from build123d import *

# Parameters (mm, degrees)
F0_W     = 47.625
F0_H     = 19.05
F1_DEPTH = 63.5
F0_W_2   = 25.4
F2_DEPTH = 25.4
F3_DEPTH = 7.9375


# Not quite as in the source:
# - a feature of the source that left no trace in its solid (it failed there, or was rolled back) is left out


with BuildPart() as f1:
    # F0 (on Front) → F1 (new body, symmetric)
    with BuildSketch(Plane.XZ):
        with Locations((-23.8125, 0)):
            Rectangle(F0_W, F0_H)
        Polygon((28.575, 9.525), (0, 9.525), (0, -9.525), (47.625, -9.525), (47.625, 9.525), align=None)
    extrude(amount=F1_DEPTH, both=True)

    # F0 (on Front) → F2 (join, symmetric)
    with BuildSketch(Plane.XZ):
        with BuildLine():
            add(Edge.make_bspline(
                [(63.5, 61.9252), (63.391502904, 61.9248401337), (63.2819047305, 61.9243249441), (63.1712168671, 61.9236523874)],
                knots=[0, 0, 0, 0, 0.5232436579, 0.5232436579, 0.5232436579, 0.5232436579], degree=3))
            ThreePointArc((63.1712168671, 61.9236523874), (38.6883255712, 51.5793870704), (28.575, 27.0002))
            Line((28.575, 27.0002), (28.575, 9.525))
            Line((28.575, 9.525), (47.625, 9.525))
            Line((47.625, 9.525), (47.625, 27.0002))
            ThreePointArc((47.625, 27.0002), (52.2746798487, 38.2255201513), (63.5, 42.8752))
            Line((63.5, 42.8752), (66.675, 42.8752))
            Line((66.675, 42.8752), (66.675, 61.9252))
            Line((66.675, 61.9252), (63.5, 61.9252))
        make_face()
        with Locations((79.375, 52.4002)):
            Rectangle(F0_W_2, F0_H)
    extrude(amount=F2_DEPTH, both=True)

    # F0 (on Front) → F3 (join, symmetric)
    with BuildSketch(Plane.XZ):
        with BuildLine():
            add(Edge.make_bspline(
                [(63.1712168671, 61.9236523874), (37.2919174266, 61.7664057285), (-48.1546851166, 53.0067745419), (-47.625, 9.525)],
                knots=[0.5232436579, 0.5232436579, 0.5232436579, 0.5232436579, 122.8598656398, 122.8598656398, 122.8598656398, 122.8598656398], degree=3))
            Line((-47.625, 9.525), (0, 9.525))
            Line((0, 9.525), (28.575, 9.525))
            Line((28.575, 9.525), (28.575, 27.0002))
            ThreePointArc((28.575, 27.0002), (38.6883255712, 51.5793870704), (63.1712168671, 61.9236523874))
        make_face()
    extrude(amount=F3_DEPTH, both=True)

    # F0 (on Front) → F4 (revolve)
    with BuildSketch(Plane.XZ):
        Polygon((92.075, 66.675), (92.075, 61.9252), (92.075, 42.8752), (92.075, 34.925), (117.475, 34.925), (117.475, 66.675), align=None)
    revolve(axis=Axis((92.075, 0, 50.8), (0, 0, -1)))


solid = f1.part
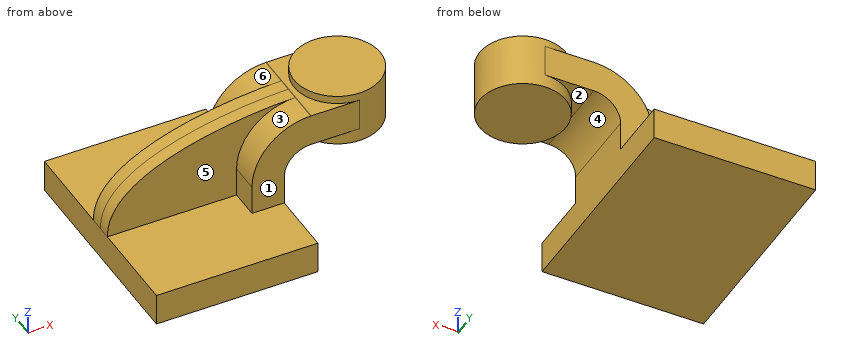
For this review, take the finished solid that the model builds, in its own axes (mm). Face numbers are marked on the shaded views. A direction names the side the tool comes from. Give positions to 0.01 mm unless a question says otherwise; leave off trailing zeros. Order: outer loops, then holes, each group sorted by start corner. A loop starts at its lowest first (then second) coordinate and runs counter-clockwise, first axis right, second up. Notation, with made-up numbers: (-35, 13.25) -> (24, 13.25) arc R20 ccw to (24, 51.25) -> close; hole circle Ø11 at (-16, -30.75). An arc over 180 degrees is marked (long way). Write item = value, one per line.
1) To check wall thickness, follow L1, parallel to X at y = 2, z = 6 (3 decimals); L2, parallel to Y at x = 41, z = 51; L3, parallel to Y at x = 9, z = 13. State the ranges of each line that lie inside material, in increasing order. Write a range as from..to.
Findings:
L1 = -47.625..47.625
L2 = -25.4..25.4
L3 = -7.94..7.94
2) Insertion check: pin 1 (19 mm diameter, centred on y = -17, z = 20.5, fed in from -X); pin 2 (8.5 mm diameter, centred on y = 19.5, z = 15, fed in from -X) (3 decimals); pin 3 (8 mm diameter, centred on x = 9, z = 39, fed in from +Y). Each pin has a flat end and moves straight along its axis. Give the tip position at first contact, or say it passes through.
Findings:
pin_1 = -46.66
pin_2 = 28.575
pin_3 = 7.94
3) Draft analysis for pull direction X (two halves, no side actions). For the marked faces 1, 2 and 3, state which applies: pulls with the +X half, pulls with the -X half, needs draft (parallel to the pull), parting line crosses it, or undercut.
Findings:
face_1 = needs draft
face_2 = undercut
face_3 = pulls with the -X half
4) For the marked faces 4, 5 and 6, list the 3-axis set-ups (+Z, -Z, +X, -X, +Y, -Y) from which the entire face can be reached by the end or side of a thin tool; tool diameter is ignored.
Findings:
face_4 = -Z, +Y, -Y
face_5 = +Z, -X, -Y
face_6 = +Z, -X, +Y
5) We need section A-A, the plane y = -29. Give the boundary of the cut face in (x, z) (3 decimals), and give its area (3 significant figures).
Findings:
outline = (-47.625, -9.525) -> (47.625, -9.525) -> (47.625, 9.525) -> (-47.625, 9.525) -> close
area = 1,810 mm^2
